Verification items for the finished model (mm, model axes). A direction names the side the tool comes from. Round coordinates to 2 decimals unless told otherwise and drop trailing zeros. Loops run counter-clockwise (first coordinate to the right, second up) from the corner with the lowest first, then second, coordinate; pieces in that order, holes last. Notation, with made-up numbers: (-24.5, 21) -> (18.5, 21) arc R27 ccw to (18.5, 39) -> close; hole circle Ø4 at (46.25, 17.25). An arc over 180 degrees is marked (long way). Use a Markdown table: item, result. Add a question column.
Autodesk Inventor part; units mm, degrees
ref_plane "XZ Plane" through (0, 0, 0) normal (0, 1, 0) x (-1, 0, 0)
ref_plane "XY Plane" through (0, 0, 0) normal (0, 0, 1) x (1, 0, 0)
sketch "スケッチ1" plane through (0, 0, 0) normal (0, 1, 0) x (-1, 0, 0)
  line L0 (14, -5) -> (-14, -5)
  line L1 (-14, -5) -> (-14, 5)
  line L2 (-14, 5) -> (14, 5)
  line L3 (14, 5) -> (14, -5)
  line L4 (-14, 5) -> (14, -5) construction
  line L5 (14, 5) -> (-14, -5) construction
  point P0 (0, 0)
  point P1 (0, 0)
  dimension "d1" = 10
  dimension "d13" = 14
extrude "押し出し1" add sketch "スケッチ1" along normal blind 1.6
sketch "スケッチ3" plane through (0, 1.6, 0) normal (0, 1, 0) x (1, 0, 0)
  line L0 (14, -5) -> (14, 5)
  line L1 (14, 5) -> (10, 5)
  line L2 (10, 5) -> (10, 3)
  line L3 (10, 3) -> (14, 3)
  line L4 (14, 3) -> (14, 5)
  line L5 (-12.25, 0) -> (12.25, 0)
  line L6 (10, -5) -> (10, -3)
  line L7 (10, -3) -> (14, -3)
  line L8 (14, -5) -> (10, -5)
  line L9 (14, -3) -> (14, -5)
  point P0 (0, 0)
  dimension "d16" = 4
  dimension "d17" = 2
extrude "押し出し2" cut sketch "スケッチ3" against normal blind 10
sketch "スケッチ4" plane through (0, 1.6, 0) normal (0, 1, 0) x (1, 0, 0)
  line L0 (10, 3) -> (10, 5)
  line L1 (10, -5) -> (10, -3)
  line L2 (10, 3) -> (10, -3)
  line L3 (10, 0) -> (14, 0)
  line L4 (14, -3) -> (14, 3)
  line L5 (-14, 5) -> (-14, -5)
  line L6 (-14, 0) -> (-12, 0)
  point P0 (0, 0)
  point P1 (12, 0)
  dimension "d27" = 2
hole "穴2" at (12, 1.6, 0) at (-12, 1.6, 0) direction (0, -1, 0) diameter 2.4 end through all
sketch "スケッチ7" plane through (0, 0, 0) normal (0, -1, 0) x (1, 0, 0)
  line L0 (75.7308, 106.5202) -> (76.0585, -99.7224)
  line L1 (75.7308, 106.5202) -> (76.0585, -99.7224)
  line L2 (0, 147.7687) -> (0, -140.9709)
  line L3 (75.7308, 106.5202) -> (76.0585, -99.7224)
  line L4 (14, 3) -> (14, -3)
  point P0 (0, 0)
  point P1 (6.4022, -1.407)
  point P2 (6.4022, -1.407)
  point P3 (-4, 0.784)
  dimension "d28" = 69.5
  dimension "d29" = 7.5978
  dimension "d31" = 18
  dimension "d32" = 79.8987
properties part number "SideSensorCircuit"
1) Release check for a two-part mould opening along X. For faces 1 (the face through (14, 1, 0)), 2 (the face through (12, 1, -3)), 3 (the face through (-10.83, 0.79, -0.26)) record: released by +X, released by -X, zero draft, split by the parting line, or undercut.
2) Sectioned sample at C-C on x = -12. Enter the section's corners in (y, z), then the cut area to 3 significant figures.
3) Sectioned sample at B-B on z = 0. Enter the section's corners in (x, y).
4) Thickness scan on line 1 (X direction, y = 0.55, z = 0); line 2 (Z direction, x = 12, y = 0.65); line 3 (X direction, y = 0.35, z = -1). Record the ranges inside material, lowest first.
5) Sectioned sample at D-D on x = 12. Enter the section's corners in (y, z).
6) Access from +Z, -Z, +X, -X, +Y, -Y to the whole of each face (thin tool, end or side, straight path). Record for faces 4 (the face through (10, 1, -4)), 5 (the face through (-14, 1, 0)), 6 (the face through (10, 1, 4)).
7) Go/stop test with flat-tipped pins: pin 1 (0.5 mm diameter, centred on y = 0.5, z = -4, fed in from +X); pin 2 (4 mm diameter, centred on x = 12, z = 0, fed in from -Y); pin 3 (0.5 mm diameter, centred on x = 11, y = 1, fed in from -Z). Record where each tip stops, or that it passes through.
8) Sectioned sample at A-A on y = 0.65. Enter the section's corners in (x, z), then the cut area to 3 significant figures.
Geometry results:
| question | item | result |
|---|---|---|
| 1 | face 1 | released by +X |
| 1 | face 2 | zero draft |
| 1 | face 3 | undercut |
| 2 | outline | (0, -5) -> (1.6, -5) -> (1.6, -1.2) -> (0, -1.2) -> close; (0, 1.2) -> (1.6, 1.2) -> (1.6, 5) -> (0, 5) -> close |
| 2 | area | 12.2 mm^2 |
| 3 | outline | (-14, 0) -> (-13.2, 0) -> (-13.2, 1.6) -> (-14, 1.6) -> close; (-10.8, 0) -> (10.8, 0) -> (10.8, 1.6) -> (-10.8, 1.6) -> close; (13.2, 0) -> (14, 0) -> (14, 1.6) -> (13.2, 1.6) -> close |
| 4 | line 1 | -14 to -13.2, -10.8 to 10.8, 13.2 to 14 |
| 4 | line 2 | -3 to -1.2, 1.2 to 3 |
| 4 | line 3 | -14 to -12.66, -11.34 to 11.34, 12.66 to 14 |
| 5 | outline | (0, -3) -> (1.6, -3) -> (1.6, -1.2) -> (0, -1.2) -> close; (0, 1.2) -> (1.6, 1.2) -> (1.6, 3) -> (0, 3) -> close |
| 6 | face 4 | -Z, +X, +Y, -Y |
| 6 | face 5 | +Z, -Z, -X, +Y, -Y |
| 6 | face 6 | +Z, +X, +Y, -Y |
| 7 | pin 1 | x = 10 |
| 7 | pin 2 | y = 0 |
| 7 | pin 3 | z = -3 |
| 8 | outline | (-14, -5) -> (10, -5) -> (10, -3) -> (14, -3) -> (14, 3) -> (10, 3) -> (10, 5) -> (-14, 5) -> close; hole circle Ø2.4 at (-12, 0); hole circle Ø2.4 at (12, 0) |
| 8 | area | 255 mm^2 |
